The figure shows three views and two pictorial views of one solid part (mm, origin at its lowest corner). Answer the questions. A direction names the side the tool comes from. Coordinates: 2 decimals unless noted, no trailing zeros. Loops run counter-clockwise (first coordinate to the right, second up) from the corner with the lowest first, then second, coordinate; pieces in that order, holes last. Notation, with made-up numbers: (-22, 11) -> (-15, 11) arc R3 cw to (-15, 16) -> close; hole circle Ø11 at (-37, 4). An arc over 180 degrees is marked (long way). Use a Markdown table: item, result. Add a question column.
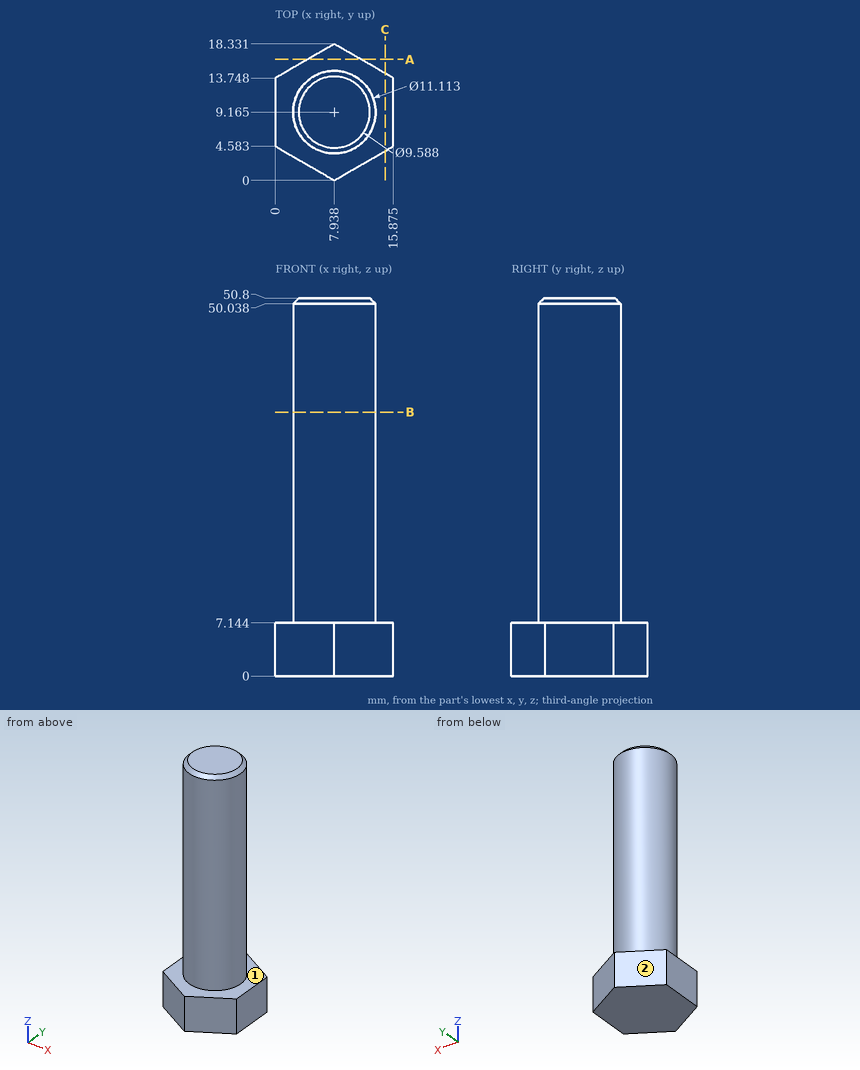
Item 1: Section B-B (z = 35.5) is taken. Determine the outline of the cut face in (x, y) (1 decimal).
Item 2: Given pin 1 (4 mm diameter, centred on x = 11, z = 20, fed in from -Y); pin 2 (1.5 mm diameter, centred on x = 12, z = 11.5, fed in from -Y) (1 decimal); pin 3 (2 mm diameter, centred on x = 13, z = 15, fed in from -Y) (1 decimal), each flat-ended and moving along its own axis, determine where each tip first touches the part or whether it passes through.
Item 3: For the marked faces 1 and 2, determine the directions among +Z, -Z, +X, -X, +Y, -Y from which every point of the face is accessible in a straight line to the end or side of a thin tool.
Item 4: Section C-C (x = 14.75) is taken. Determine the outline of the cut face in (y, z).
Item 5: Find the intervals of material crossed by probe 1 along Z at (x, y) = (15, 6); probe 2 along X at (y, z) = (5.75, 29) (1 decimal); probe 3 along Z at (x, y) = (12, 11.75), in increasing order.
Item 6: Section A-A (y = 16.25) is taken. Determine the outline of the cut face in (x, z).
Output:
| question | item | result |
|---|---|---|
| 1 | outline | circle Ø11.1 at (7.9, 9.2) |
| 2 | pin 1 | stops at y = 3.71 |
| 2 | pin 2 | stops at y = 4.7 |
| 2 | pin 3 | stops at y = 5.4 |
| 3 | face 1 | +Z |
| 3 | face 2 | +Z, -Z, -X, +Y |
| 4 | outline | (3.93, 0) -> (14.4, 0) -> (14.4, 7.14) -> (3.93, 7.14) -> close |
| 5 | probe 1 | z = 0 to 7.14 |
| 5 | probe 2 | x = 3.6 to 12.3 |
| 5 | probe 3 | z = 0 to 50.78 |
| 6 | outline | (4.33, 0) -> (11.54, 0) -> (11.54, 7.14) -> (4.33, 7.14) -> close |
